Verification items for the finished model (mm, model axes). A direction names the side the tool comes from. Round coordinates to 2 decimals unless told otherwise and drop trailing zeros. Loops run counter-clockwise (first coordinate to the right, second up) from the corner with the lowest first, then second, coordinate; pieces in that order, holes last. Notation, with made-up numbers: (73.5, 50) -> (111.5, 50) arc R29 ccw to (111.5, 83) -> close; hole circle Ø4 at (-34, 14.5). An arc over 180 degrees is marked (long way). Write item = value, one per line.
```python
from build123d import *

# Parameters (mm, degrees)
SKETCH1_R           = 10
BOSS_EXTRUDE1_DEPTH = 20


with BuildPart() as part:
    # Sketch1 → Boss-Extrude1 (new body)
    with BuildSketch(Plane.XY):
        with BuildLine():
            Line((-75, 0), (75, 0))
            Line((75, 0), (75, 20))
            ThreePointArc((75, 20), (72.071067812, 27.071067812), (65, 30))
            Line((65, 30), (35, 30))
            ThreePointArc((35, 30), (27.928932188, 32.928932188), (25, 40))
            Line((25, 40), (25, 90))
            Line((25, 90), (15, 100))
            Line((15, 100), (-15, 100))
            Line((-15, 100), (-25, 90))
            Line((-25, 90), (-25, 40))
            ThreePointArc((-25, 40), (-27.928932188, 32.928932188), (-35, 30))
            Line((-35, 30), (-65, 30))
            ThreePointArc((-65, 30), (-72.071067812, 27.071067812), (-75, 20))
            Line((-75, 20), (-75, 0))
        make_face()
        with Locations((-50, 15)):
            Circle(SKETCH1_R, mode=Mode.SUBTRACT)
        with Locations(Location((50, 15, 0), (0, 0, 180))):
            Circle(SKETCH1_R, mode=Mode.SUBTRACT)
    extrude(amount=BOSS_EXTRUDE1_DEPTH)


solid = part.part
```
(1) Draft check along Y on faces 1 (the face through (-20, 95, 10)), 2 (the face through (-60, 15, 10)), 3 (the face through (60, 15, 10)), 4 (the face through (-75, 10, 10)). Enter one of: released by +Y, released by -Y, zero draft, split by the parting line, or undercut.
Filled sheet:
face_1 = released by +Y
face_2 = undercut
face_3 = undercut
face_4 = zero draft
(2) Sectioned sample at B-B, the plane x = 50. Record the cut outline in (y, z).
Filled sheet:
outline = (0, 0) -> (5, 0) -> (5, 20) -> (0, 20) -> close; (25, 0) -> (30, 0) -> (30, 20) -> (25, 20) -> close
(3) Set-up check for faces 5 (the face through (75, 10, 10)), 6 (the face through (-50, 30, 10)), 7 (the face through (50, 30, 10)): record each of +Z, -Z, +X, -X, +Y, -Y from which the full face is reachable in a straight line by a thin tool's end or side.
Filled sheet:
face_5 = +Z, -Z, +X, +Y, -Y
face_6 = +Z, -Z, -X, +Y
face_7 = +Z, -Z, +X, +Y
(4) Sectioned sample at D-D, the plane y = 68. Record the cut outline in (x, z), and give its area (3 significant figures).
Filled sheet:
outline = (-25, 0) -> (25, 0) -> (25, 20) -> (-25, 20) -> close
area = 1,000 mm2
(5) Material ranges on probe 1 along Y at (x, z) = (50, 12.5); probe 2 along X at (y, z) = (6, 14.5); probe 3 along Y at (x, z) = (-64.5, 7.25), recorded low to high. Write a range as from..to.
Filled sheet:
probe_1 = 0..5, 25..30
probe_2 = -75..-54.36, -45.64..45.64, 54.36..75
probe_3 = 0..30
(6) Go/stop test with flat-tipped pins: pin 1 Ø3 at (y, z) = (77.5, 9.5) entering from -X; pin 2 Ø10 at (y, z) = (43.5, 8.5) entering from -X; pin 3 Ø1 at (y, z) = (34.5, 8) entering from +X. Record where each tip stops, or that it passes through.
Filled sheet:
pin_1 = -25
pin_2 = -25.11
pin_3 = 27
(7) Sectioned sample at C-C, the plane z = 1.5. Record the cut outline in (x, y), and give its area (3 significant figures).
Filled sheet:
outline = (-75, 0) -> (75, 0) -> (75, 20) arc R10 ccw to (65, 30) -> (35, 30) arc R10 cw to (25, 40) -> (25, 90) -> (15, 100) -> (-15, 100) -> (-25, 90) -> (-25, 40) arc R10 cw to (-35, 30) -> (-65, 30) arc R10 ccw to (-75, 20) -> close; hole circle Ø20 at (-50, 15); hole circle Ø20 at (50, 15)
area = 7,270 mm2
(8) Sectioned sample at A-A, the plane y = 15. Record the cut outline in (x, z), and give its area (3 significant figures).
Filled sheet:
outline = (-75, 0) -> (-60, 0) -> (-60, 20) -> (-75, 20) -> close; (-40, 0) -> (40, 0) -> (40, 20) -> (-40, 20) -> close; (60, 0) -> (75, 0) -> (75, 20) -> (60, 20) -> close
area = 2,200 mm2
